The model under review builds one solid part; all positions refer to its coordinate system, in mm. A direction names the side the tool comes from. Coordinates: 2 decimals unless noted, no trailing zeros. Write each loop counter-clockwise with the first axis right and the second up, starting at its lowest first coordinate (ties: lowest second). Pieces come first, ordered by that corner, then holes. Notation, with made-up numbers: (71, 8) -> (95, 8) arc R17 cw to (95, 28) -> close; hole circle Ø6 at (40, -31). An arc over 180 degrees is marked (long way). Put each result on its own line as item: value. Start each with the question number.
Autodesk Inventor part; units mm, degrees
ref_plane "YZ Plane" through (0, 0, 0) normal (1, 0, 0) x (0, 1, 0)
ref_plane "XZ Plane" through (0, 0, 0) normal (0, 1, 0) x (-1, 0, 0)
ref_plane "XY Plane" through (0, 0, 0) normal (0, 0, 1) x (1, 0, 0)
sketch "草图1" plane through (0, 0, 0) normal (0, 1, 0) x (-1, 0, 0)
  circle A0 centre (0, 0) radius 6.5
  circle A1 centre (0, 0) radius 3
  dimension "d0" = 13
  dimension "d1" = 6
extrude "拉伸1" add sketch "草图1" along normal blind 4
sketch "草图2" plane through (0, 4, 0) normal (0, 1, 0) x (1, 0, 0)
  circle A0 centre (0, 0) radius 3
  circle A1 centre (0, 0) radius 6.5
  circle A2 centre (0, 0) radius 3.75
  circle A3 centre (0, 0) radius 5.75
  dimension "d4" = 11.5
  dimension "d5" = 7.5
extrude "拉伸2" cut sketch "草图2" against normal blind 0.5 contours A3
sketch "草图3" plane through (0, 0, 0) normal (0, -1, 0) x (1, 0, 0)
  circle A0 centre (0, 0) radius 3.75
  circle A1 centre (0, 0) radius 5.75
extrude "拉伸3" cut sketch "草图3" against normal blind 0.5
properties part number "bearing_6_13_5"
1. The part is to be moulded in two halves that separate along X. For faces 1 (the cylindrical face through (3, 2, 0)), 2 (the cylindrical face through (5.158, 1.972, 3.955)), 3 (the flat face through (-1, 4, 3)), 4 (the flat face through (0, 0.5, -4)), say which applies: released by +X, released by -X, zero draft, split by the parting line, or undercut.
2. Consider section B-B on z = 0. State the section outline as (x, y) points, then the cut area to 3 significant figures.
3. Insertion check: P1, Ø1.5, axis at x = -1.5, y = 2, coming from the -Z side; P2, Ø1, axis at x = 1, y = 1.5, coming from the +Z side. Each pin has a flat end and moves straight along its axis. Give the tip position at first contact, or say it passes through.
4. Tool access review of faces 5 (the cylindrical face through (-3.746, 0.246, 0.165)), 6 (the cylindrical face through (-3.746, 3.754, -0.165)), 7 (the flat face through (-1, 0, 3)): name each direction out of +Z, -Z, +X, -X, +Y, -Y from which nothing blocks a thin tool from reaching the whole face with its end or side.
5. Wall thickness on line 1 (Z direction, x = 0, y = 0.15); line 2 (Z direction, x = -2, y = 3.6); line 3 (X direction, y = 0.4, z = -3.25): over which ranges is each line inside the solid? List them lowest first. Write a range as from..to.
6. Consider section C-C on y = 0.3. State the section outline as (x, z) points, then the cut area to 3 significant figures.
7. Consider section D-D on y = 2.8. State the section outline as (x, z) points.
8. Consider section A-A on x = 0. State the section outline as (y, z) points, then the cut area to 3 significant figures.
Output values:
1. face 1: undercut
1. face 2: split by the parting line
1. face 3: zero draft
1. face 4: undercut
2. outline: (-6.5, 0) -> (-5.75, 0) -> (-5.75, 0.5) -> (-3.75, 0.5) -> (-3.75, 0) -> (-3, 0) -> (-3, 4) -> (-3.75, 4) -> (-3.75, 3.5) -> (-5.75, 3.5) -> (-5.75, 4) -> (-6.5, 4) -> close; (3, 0) -> (3.75, 0) -> (3.75, 0.5) -> (5.75, 0.5) -> (5.75, 0) -> (6.5, 0) -> (6.5, 4) -> (5.75, 4) -> (5.75, 3.5) -> (3.75, 3.5) -> (3.75, 4) -> (3, 4) -> close
2. area: 24.0 mm^2
3. P1: stops at z = -6.46
3. P2: stops at z = 6.48
4. face 5: -Y
4. face 6: +Y
4. face 7: +Z, -Z, +X, -X, -Y
5. line 1: z = -6.5..-5.75, -3.75..-3, 3..3.75, 5.75..6.5
5. line 2: z = -6.18..-5.39, -3.17..-2.24, 2.24..3.17, 5.39..6.18
5. line 3: x = -5.63..-4.74, -1.87..1.87, 4.74..5.63
6. outline: circle Ø13 at (0, 0); circle Ø7.5 at (0, 0); hole circle Ø11.5 at (0, 0); hole circle Ø6 at (0, 0)
6. area: 44.8 mm^2
7. outline: circle Ø13 at (0, 0); hole circle Ø6 at (0, 0)
8. outline: (0, -6.5) -> (4, -6.5) -> (4, -5.75) -> (3.5, -5.75) -> (3.5, -3.75) -> (4, -3.75) -> (4, -3) -> (0, -3) -> (0, -3.75) -> (0.5, -3.75) -> (0.5, -5.75) -> (0, -5.75) -> close; (0, 3) -> (4, 3) -> (4, 3.75) -> (3.5, 3.75) -> (3.5, 5.75) -> (4, 5.75) -> (4, 6.5) -> (0, 6.5) -> (0, 5.75) -> (0.5, 5.75) -> (0.5, 3.75) -> (0, 3.75) -> close
8. area: 24.0 mm^2
